```python
from build123d import *

# Parameters (mm, degrees)
F0_W     = 150
F0_H     = 20
F1_DEPTH = 2.5
F3_D     = 7.5
F4_R     = 9.99999
F5_W     = 2.5
F5_H     = 5
F6_DEPTH = 30


# Not quite as in the source:
# - a fillet or chamfer is up to 0.001 mm smaller than in the source, because OpenCascade refuses the exact size


with BuildPart() as f1:
    # F0 (on Top) → F1 (new body)
    with BuildSketch(Plane.XY):
        Rectangle(F0_W, F0_H)
    extrude(amount=F1_DEPTH)

    # F3 (through all)
    with Locations(Plane.XY.offset(2.5)):
        with Locations((-65, 0)):
            Hole(F3_D / 2)

    # F4 (radius 10 in the source; OpenCascade refuses exactly that, so slightly less here)
    f4_edges = [f1.edges().sort_by_distance(p)[0] for p in [
        (-75, -10, 1.25),
        (-75, 10, 1.25),
    ]]
    fillet(f4_edges, radius=F4_R)

    # F5 (on face) → F6 (join)
    with BuildSketch(Plane.YZ.offset(75)):
        with BuildLine():
            Line((-10, 0), (-10, 2.5))
            ThreePointArc((-10, 2.5), (-12.4748737342, 1.4748737342), (-13.5, -1))
            Line((-13.5, -1), (-11, -1))
            ThreePointArc((-11, -1), (-10.7071067812, -0.2928932188), (-10, 0))
        make_face()
        with Locations((-12.25, -3.5)):
            Rectangle(F5_W, F5_H)
    extrude(amount=-F6_DEPTH)


solid = f1.part
```
Check sheet for the modelled part. Datum: model origin and axes. Units: mm. A direction names the side the tool comes from. Coordinates: 2 decimals unless noted, no trailing zeros. Write each loop counter-clockwise with the first axis right and the second up, starting at its lowest first coordinate (ties: lowest second). Pieces come first, ordered by that corner, then holes. Notation, with made-up numbers: (13.5, 5.5) -> (47.5, 5.5) arc R35 ccw to (47.5, 40.5) -> close; hole circle Ø7 at (-12, -30.75). An arc over 180 degrees is marked (long way). Use a Markdown table: item, result.
1. Sectioned sample at C-C (z = -4). Enter the section's corners in (x, y), plus the area to 3 significant figures.
Reported:
| item | result |
|---|---|
| outline | (45, -13.5) -> (75, -13.5) -> (75, -11) -> (45, -11) -> close |
| area | 75.0 mm2 |
2. Sectioned sample at B-B (y = -2.25). Enter the section's corners in (x, z), plus the area to 3 significant figures.
Reported:
| item | result |
|---|---|
| outline | (-74.74, 0) -> (-68, 0) -> (-68, 2.5) -> (-74.74, 2.5) -> close; (-62, 0) -> (75, 0) -> (75, 2.5) -> (-62, 2.5) -> close |
| area | 359 mm2 |
3. Scan lines: line 1 along Y through (x, z) = (-65, 1.3); line 2 along Z through (x, y) = (58.5, -5.5); line 3 along Y through (x, z) = (42, 0.75). Record each from-to range of solid material in increasing order.
Reported:
| item | result |
|---|---|
| line 1 | y = -10 to -3.75, 3.75 to 10 |
| line 2 | z = 0 to 2.5 |
| line 3 | y = -10 to 10 |
4. Release check for a two-part mould opening along Y. For faces 1 (the flat face through (60, -13.5, -4)), 2 (the flat face through (4, 10, 1)), 3 (the flat face through (-1, 0, 2.5)), 4 (the cylindrical face through (-68.464, -1.436, 1.232)) record: pulls with the +Y half, pulls with the -Y half, needs draft (parallel to the pull), parting line crosses it, or undercut.
Reported:
| item | result |
|---|---|
| face 1 | pulls with the -Y half |
| face 2 | pulls with the +Y half |
| face 3 | needs draft |
| face 4 | undercut |
5. Tool access check on faces 5 (the flat face through (45, -12, -2)), 6 (the flat face through (-1, 0, 0)), 7 (the flat face through (60, -12, -6)). Record the directions out of +Z, -Z, +X, -X, +Y, -Y that give a thin tool (end or side, any length) a straight path to the whole face; none if there is none.
Reported:
| item | result |
|---|---|
| face 5 | +Z, -Z, -X, -Y |
| face 6 | -Z, +X, -X, +Y |
| face 7 | -Z, +X, -X, +Y, -Y |
6. Sectioned sample at D-D (x = 28.5). Enter the section's corners in (y, z).
Reported:
| item | result |
|---|---|
| outline | (-10, 0) -> (10, 0) -> (10, 2.5) -> (-10, 2.5) -> close |
7. Go/stop test with flat-tipped pins: pin 1 Ø0.8 at (x, z) = (12.5, 1) entering from -Y; pin 2 Ø10 at (x, y) = (-65, 0) entering from -Z; pin 3 Ø1.8 at (y, z) = (-12.5, -2) entering from -X. Record where each tip stops, or that it passes through.
Reported:
| item | result |
|---|---|
| pin 1 | stops at y = -10 |
| pin 2 | stops at z = 0 |
| pin 3 | stops at x = 45 |
8. Sectioned sample at A-A (x = 61). Enter the section's corners in (y, z), plus the area to 3 significant figures.
Reported:
| item | result |
|---|---|
| outline | (-13.5, -6) -> (-11, -6) -> (-11, -1) arc R1 cw to (-10, 0) -> (10, 0) -> (10, 2.5) -> (-10, 2.5) arc R3.5 ccw to (-13.5, -1) -> close |
| area | 71.3 mm2 |
